Geometry check sheet. Reference: the model listing, model coordinates, mm. Coordinates: 2 decimals unless noted, no trailing zeros. Order: outer loops, then holes, each group sorted by start corner. A loop starts at its lowest first (then second) coordinate and runs counter-clockwise, first axis right, second up. Notation, with made-up numbers: (75, 69.25) - (106, 69.25) arc R14 ccw to (106, 83.25) - close; hole circle Ø5 at (69.5, 72). An arc over 180 degrees is marked (long way). Put each result on its own line as item: value.
from build123d import *

# Parameters (mm, degrees)
F0_R     = 10
F1_DEPTH = 2
F2_R     = 20


with BuildPart() as f1:
    # F0 (on Top) → F1 (new body)
    with BuildSketch(Plane.XY):
        with BuildLine():
            Line((0, 0), (-45, 0))
            Line((-45, 0), (-37.5, -50))
            Line((-37.5, -50), (0, -50))
            Line((0, -50), (0, -35))
            ThreePointArc((0, -35), (-10, -25), (0, -15))
            Line((0, -15), (0, 0))
        make_face()
        with Locations((-22, -25)):
            Circle(F0_R, mode=Mode.SUBTRACT)
        with BuildLine():
            Line((45, 0), (0, 0))
            Line((0, 0), (0, -15))
            ThreePointArc((0, -15), (7.071068, -17.928932), (10, -25))
            ThreePointArc((10, -25), (7.071068, -32.071068), (0, -35))
            Line((0, -35), (0, -50))
            Line((0, -50), (37.5, -50))
            Line((37.5, -50), (45, 0))
        make_face()
        with Locations((22, -25)):
            Circle(F0_R, mode=Mode.SUBTRACT)
    extrude(amount=F1_DEPTH)

    # F2
    f2_edges = [f1.edges().sort_by_distance(p)[0] for p in [
        (-37.5, -50, 1),
        (37.5, -50, 1),
        (45, 0, 1),
        (-45, 0, 1),
    ]]
    fillet(f2_edges, radius=F2_R)


solid = f1.part
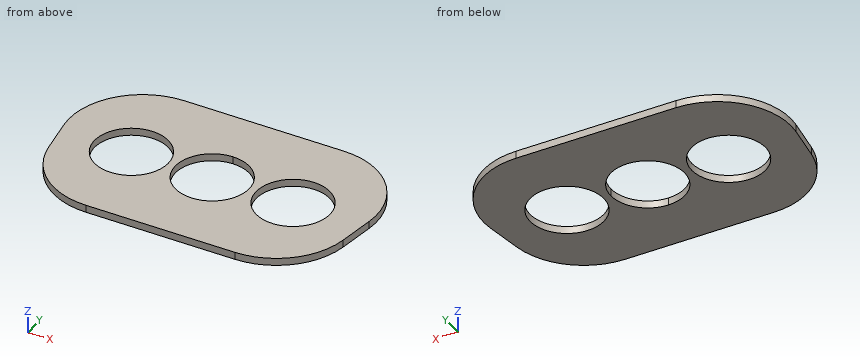
Q1. Section check D-D on x = 29. Record the boundary of the cut face in (y, z).
Answer block:
outline: (-48, 0) - (-32.14, 0) - (-32.14, 2) - (-48, 2) - close; (-17.86, 0) - (-1.35, 0) - (-1.35, 2) - (-17.86, 2) - close
Q2. Section check A-A on x = -27. Record the boundary of the cut face in (y, z), then the cut area to 3 significant figures.
Answer block:
outline: (-48.84, 0) - (-33.66, 0) - (-33.66, 2) - (-48.84, 2) - close; (-16.34, 0) - (-0.69, 0) - (-0.69, 2) - (-16.34, 2) - close
area: 61.6 mm^2
Q3. Depth check by flat-ended pin: pin 1 Ø18 at (x, y) = (-22, -25) entering from -Z. Enter the tip coordinate at first touch or a pass-through.
Answer block:
pin 1: passes through
Q4. Section check B-B on z = 1.35. Record the boundary of the cut face in (x, y).
Answer block:
outline: (-41.55, -22.97) - (-40.05, -32.97) arc R20 ccw to (-20.28, -50) - (20.28, -50) arc R20 ccw to (40.05, -32.97) - (41.55, -22.97) arc R20 ccw to (21.78, 0) - (-21.78, 0) arc R20 ccw to start; hole circle Ø20 at (-22, -25); hole (0, -15) arc R10 ccw (long way) to (10, -25) arc R10 ccw to start; hole circle Ø20 at (22, -25)
Q5. Thickness scan on L1, parallel to X at y = -19, z = 0.2; L2, parallel to X at y = -28, z = 0.8; L3, parallel to Y at x = -22, z = 0.8. Record the ranges inside material, lowest first. Write a range as [from, to].
Answer block:
L1: x = [-41.75, -30], [-14, -8], [8, 14], [30, 41.75]
L2: x = [-40.8, -31.54], [-12.46, -9.54], [9.54, 12.46], [31.54, 40.8]
L3: y = [-49.93, -35], [-15, 0]
Q6. Section check C-C on y = -28. Record the boundary of the cut face in (x, z), then the cut area to 3 significant figures.
Answer block:
outline: (-40.8, 0) - (-31.54, 0) - (-31.54, 2) - (-40.8, 2) - close; (-12.46, 0) - (-9.54, 0) - (-9.54, 2) - (-12.46, 2) - close; (9.54, 0) - (12.46, 0) - (12.46, 2) - (9.54, 2) - close; (31.54, 0) - (40.8, 0) - (40.8, 2) - (31.54, 2) - close
area: 48.7 mm^2
